Part model, mm, in its own coordinate system. Round coordinates to 2 decimals unless told otherwise and drop trailing zeros. Loops run counter-clockwise (first coordinate to the right, second up) from the corner with the lowest first, then second, coordinate; pieces in that order, holes last.
(1) Cut at C-C on y = 2. Count the separate pieces of the cut face and the enclosed holes in it, then the cut area to 3 significant figures.
(2) Cut at A-A on x = 0. List the corners of the cut face in (y, z), then the cut area to 3 significant figures.
(3) Cut at B-B on z = 0. List the corners of the cut face in (x, y), then the cut area to 3 significant figures.
(4) Flat gauge pin, fed straight in: pin 1 (3 mm diameter, centred on y = 3.5, z = -66, fed in from -X). Where does the tip first touch, or does it go through?
(5) Probe probe 1 along X at (y, z) = (2, 0); probe 2 along X at (y, z) = (5.6, 0); probe 3 along Z at (x, y) = (-44.5, 4). List the from-to ranges inside material, lowest first.
from build123d import *

# Parameters (mm, degrees)
SKETCH1_R           = 101.6
BOSS_EXTRUDE1_DEPTH = 6.35
SKETCH2_R           = 63.5
CUT_EXTRUDE1_DEPTH  = 144.824345992
CUT_EXTRUDE2_REACH  = 145.824
SKETCH3_R           = 3.175
SKETCH4_R           = 73.9394
SKETCH4_R_2         = 69.85
CUT_EXTRUDE3_DEPTH  = 2.6416
FILLET1_R           = 0.4318


with BuildPart() as part:
    # Sketch1 → Boss-Extrude1 (new body)
    with BuildSketch(Plane(origin=(0, 0, 0), x_dir=(1, 0, 0), z_dir=(0, 1, 0))):
        with Locations(Location((0, 0, 0), (0, 0, 270))):
            Circle(SKETCH1_R)
    extrude(amount=BOSS_EXTRUDE1_DEPTH)

    # Sketch2 → Cut-Extrude1 (cut, through all)
    with BuildSketch(Plane(origin=(0, 6.35, 0), x_dir=(1, 0, 0), z_dir=(0, 1, 0))):
        with Locations(Location((0, 0, 0), (0, 0, 270))):
            Circle(SKETCH2_R)
    extrude(amount=-CUT_EXTRUDE1_DEPTH, mode=Mode.SUBTRACT)

    # Sketch3 → Cut-Extrude2 (cut, up to next)
    with BuildSketch(Plane(origin=(0, 6.35, 0), x_dir=(1, 0, 0), z_dir=(0, 1, 0)), mode=Mode.PRIVATE) as cut_extrude2_sk1:
        with Locations(Location((0, 85.725, 0), (0, 0, 270))):
            Circle(SKETCH3_R)
    cut_extrude2_tool1 = extrude(cut_extrude2_sk1.sketch, amount=-CUT_EXTRUDE2_REACH, mode=Mode.PRIVATE) & part.part
    # Sketch3 → Cut-Extrude2 (cut, up to next)
    with BuildSketch(Plane(origin=(0, 6.35, 0), x_dir=(1, 0, 0), z_dir=(0, 1, 0)), mode=Mode.PRIVATE) as cut_extrude2_sk2:
        with Locations(Location((42.8625, 74.240027739, 0), (0, 0, 270))):
            Circle(SKETCH3_R)
    cut_extrude2_tool2 = extrude(cut_extrude2_sk2.sketch, amount=-CUT_EXTRUDE2_REACH, mode=Mode.PRIVATE) & part.part
    # Sketch3 → Cut-Extrude2 (cut, up to next)
    with BuildSketch(Plane(origin=(0, 6.35, 0), x_dir=(1, 0, 0), z_dir=(0, 1, 0)), mode=Mode.PRIVATE) as cut_extrude2_sk3:
        with Locations(Location((74.240027739, 42.8625, 0), (0, 0, 270))):
            Circle(SKETCH3_R)
    cut_extrude2_tool3 = extrude(cut_extrude2_sk3.sketch, amount=-CUT_EXTRUDE2_REACH, mode=Mode.PRIVATE) & part.part
    # Sketch3 → Cut-Extrude2 (cut, up to next)
    with BuildSketch(Plane(origin=(0, 6.35, 0), x_dir=(1, 0, 0), z_dir=(0, 1, 0)), mode=Mode.PRIVATE) as cut_extrude2_sk4:
        with Locations(Location((85.725, 0, 0), (0, 0, 270))):
            Circle(SKETCH3_R)
    cut_extrude2_tool4 = extrude(cut_extrude2_sk4.sketch, amount=-CUT_EXTRUDE2_REACH, mode=Mode.PRIVATE) & part.part
    # Sketch3 → Cut-Extrude2 (cut, up to next)
    with BuildSketch(Plane(origin=(0, 6.35, 0), x_dir=(1, 0, 0), z_dir=(0, 1, 0)), mode=Mode.PRIVATE) as cut_extrude2_sk5:
        with Locations(Location((74.240027739, -42.8625, 0), (0, 0, 270))):
            Circle(SKETCH3_R)
    cut_extrude2_tool5 = extrude(cut_extrude2_sk5.sketch, amount=-CUT_EXTRUDE2_REACH, mode=Mode.PRIVATE) & part.part
    # Sketch3 → Cut-Extrude2 (cut, up to next)
    with BuildSketch(Plane(origin=(0, 6.35, 0), x_dir=(1, 0, 0), z_dir=(0, 1, 0)), mode=Mode.PRIVATE) as cut_extrude2_sk6:
        with Locations(Location((42.8625, -74.240027739, 0), (0, 0, 270))):
            Circle(SKETCH3_R)
    cut_extrude2_tool6 = extrude(cut_extrude2_sk6.sketch, amount=-CUT_EXTRUDE2_REACH, mode=Mode.PRIVATE) & part.part
    # Sketch3 → Cut-Extrude2 (cut, up to next)
    with BuildSketch(Plane(origin=(0, 6.35, 0), x_dir=(1, 0, 0), z_dir=(0, 1, 0)), mode=Mode.PRIVATE) as cut_extrude2_sk7:
        with Locations(Location((0, -85.725, 0), (0, 0, 270))):
            Circle(SKETCH3_R)
    cut_extrude2_tool7 = extrude(cut_extrude2_sk7.sketch, amount=-CUT_EXTRUDE2_REACH, mode=Mode.PRIVATE) & part.part
    # Sketch3 → Cut-Extrude2 (cut, up to next)
    with BuildSketch(Plane(origin=(0, 6.35, 0), x_dir=(1, 0, 0), z_dir=(0, 1, 0)), mode=Mode.PRIVATE) as cut_extrude2_sk8:
        with Locations(Location((-42.8625, -74.240027739, 0), (0, 0, 270))):
            Circle(SKETCH3_R)
    cut_extrude2_tool8 = extrude(cut_extrude2_sk8.sketch, amount=-CUT_EXTRUDE2_REACH, mode=Mode.PRIVATE) & part.part
    # Sketch3 → Cut-Extrude2 (cut, up to next)
    with BuildSketch(Plane(origin=(0, 6.35, 0), x_dir=(1, 0, 0), z_dir=(0, 1, 0)), mode=Mode.PRIVATE) as cut_extrude2_sk9:
        with Locations(Location((-74.240027739, -42.8625, 0), (0, 0, 270))):
            Circle(SKETCH3_R)
    cut_extrude2_tool9 = extrude(cut_extrude2_sk9.sketch, amount=-CUT_EXTRUDE2_REACH, mode=Mode.PRIVATE) & part.part
    # Sketch3 → Cut-Extrude2 (cut, up to next)
    with BuildSketch(Plane(origin=(0, 6.35, 0), x_dir=(1, 0, 0), z_dir=(0, 1, 0)), mode=Mode.PRIVATE) as cut_extrude2_sk10:
        with Locations(Location((-85.725, 0, 0), (0, 0, 270))):
            Circle(SKETCH3_R)
    cut_extrude2_tool10 = extrude(cut_extrude2_sk10.sketch, amount=-CUT_EXTRUDE2_REACH, mode=Mode.PRIVATE) & part.part
    # Sketch3 → Cut-Extrude2 (cut, up to next)
    with BuildSketch(Plane(origin=(0, 6.35, 0), x_dir=(1, 0, 0), z_dir=(0, 1, 0)), mode=Mode.PRIVATE) as cut_extrude2_sk11:
        with Locations(Location((-74.240027739, 42.8625, 0), (0, 0, 270))):
            Circle(SKETCH3_R)
    cut_extrude2_tool11 = extrude(cut_extrude2_sk11.sketch, amount=-CUT_EXTRUDE2_REACH, mode=Mode.PRIVATE) & part.part
    # Sketch3 → Cut-Extrude2 (cut, up to next)
    with BuildSketch(Plane(origin=(0, 6.35, 0), x_dir=(1, 0, 0), z_dir=(0, 1, 0)), mode=Mode.PRIVATE) as cut_extrude2_sk12:
        with Locations(Location((-42.8625, 74.240027739, 0), (0, 0, 270))):
            Circle(SKETCH3_R)
    cut_extrude2_tool12 = extrude(cut_extrude2_sk12.sketch, amount=-CUT_EXTRUDE2_REACH, mode=Mode.PRIVATE) & part.part
    add(cut_extrude2_tool1.solids().sort_by_distance((0, 6.35, -85.725))[0], mode=Mode.SUBTRACT)
    add(cut_extrude2_tool2.solids().sort_by_distance((42.8625, 6.35, -74.240028))[0], mode=Mode.SUBTRACT)
    add(cut_extrude2_tool3.solids().sort_by_distance((74.240028, 6.35, -42.8625))[0], mode=Mode.SUBTRACT)
    add(cut_extrude2_tool4.solids().sort_by_distance((85.725, 6.35, 0))[0], mode=Mode.SUBTRACT)
    add(cut_extrude2_tool5.solids().sort_by_distance((74.240028, 6.35, 42.8625))[0], mode=Mode.SUBTRACT)
    add(cut_extrude2_tool6.solids().sort_by_distance((42.8625, 6.35, 74.240028))[0], mode=Mode.SUBTRACT)
    add(cut_extrude2_tool7.solids().sort_by_distance((0, 6.35, 85.725))[0], mode=Mode.SUBTRACT)
    add(cut_extrude2_tool8.solids().sort_by_distance((-42.8625, 6.35, 74.240028))[0], mode=Mode.SUBTRACT)
    add(cut_extrude2_tool9.solids().sort_by_distance((-74.240028, 6.35, 42.8625))[0], mode=Mode.SUBTRACT)
    add(cut_extrude2_tool10.solids().sort_by_distance((-85.725, 6.35, 0))[0], mode=Mode.SUBTRACT)
    add(cut_extrude2_tool11.solids().sort_by_distance((-74.240028, 6.35, -42.8625))[0], mode=Mode.SUBTRACT)
    add(cut_extrude2_tool12.solids().sort_by_distance((-42.8625, 6.35, -74.240028))[0], mode=Mode.SUBTRACT)

    # Sketch4 → Cut-Extrude3 (cut)
    with BuildSketch(Plane(origin=(0, 6.35, 0), x_dir=(1, 0, 0), z_dir=(0, 1, 0))):
        with Locations(Location((0, 0, 0), (0, 0, 270))):
            Circle(SKETCH4_R)
        with Locations(Location((0, 0, 0), (0, 0, 270))):
            Circle(SKETCH4_R_2, mode=Mode.SUBTRACT)
    extrude(amount=-CUT_EXTRUDE3_DEPTH, mode=Mode.SUBTRACT)

    # Fillet1
    fillet1_edges = [part.edges().sort_by_distance(p)[0] for p in [
        (0, 3.7084, -73.9394),
        (0, 3.7084, -69.85),
    ]]
    fillet(fillet1_edges, radius=FILLET1_R)


solid = part.part
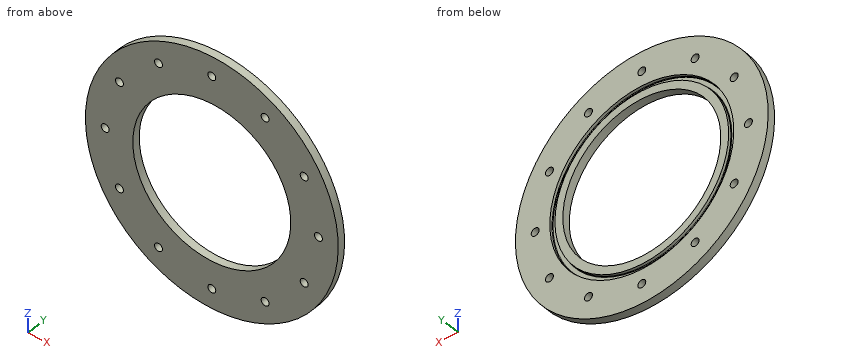
Final values:
1. separate pieces: 1
1. enclosed holes: 13
1. area: 19,400 mm2
2. outline: (0, -101.6) - (6.35, -101.6) - (6.35, -88.9) - (0, -88.9) - close; (0, -82.55) - (6.35, -82.55) - (6.35, -73.94) - (4.14, -73.94) arc R0.43 cw to (3.71, -73.51) - (3.71, -70.28) arc R0.43 cw to (4.14, -69.85) - (6.35, -69.85) - (6.35, -63.5) - (0, -63.5) - close; (0, 63.5) - (6.35, 63.5) - (6.35, 69.85) - (4.14, 69.85) arc R0.43 cw to (3.71, 70.28) - (3.71, 73.51) arc R0.43 cw to (4.14, 73.94) - (6.35, 73.94) - (6.35, 82.55) - (0, 82.55) - close; (0, 88.9) - (6.35, 88.9) - (6.35, 101.6) - (0, 101.6) - close
2. area: 382 mm2
3. outline: (-101.6, 0) - (-88.9, 0) - (-88.9, 6.35) - (-101.6, 6.35) - close; (-82.55, 0) - (-63.5, 0) - (-63.5, 6.35) - (-69.85, 6.35) - (-69.85, 4.14) arc R0.43 cw to (-70.28, 3.71) - (-73.51, 3.71) arc R0.43 cw to (-73.94, 4.14) - (-73.94, 6.35) - (-82.55, 6.35) - close; (63.5, 0) - (82.55, 0) - (82.55, 6.35) - (73.94, 6.35) - (73.94, 4.14) arc R0.43 cw to (73.51, 3.71) - (70.28, 3.71) arc R0.43 cw to (69.85, 4.14) - (69.85, 6.35) - (63.5, 6.35) - close; (88.9, 0) - (101.6, 0) - (101.6, 6.35) - (88.9, 6.35) - close
3. area: 382 mm2
4. pin 1: stops at x = -78.5
5. probe 1: x = -101.6 to -88.9, -82.55 to -63.5, 63.5 to 82.55, 88.9 to 101.6
5. probe 2: x = -101.6 to -88.9, -82.55 to -73.94, -69.85 to -63.5, 63.5 to 69.85, 73.94 to 82.55, 88.9 to 101.6
5. probe 3: z = -91.34 to -76.96, -71.52 to -59.02, -53.87 to -45.3, 45.3 to 53.87, 59.02 to 71.52, 76.96 to 91.34
